Could you check a few things on this model? Use its own coordinates, in mm. Face numbers are marked on the shaded views. Round coordinates to 2 decimals unless told otherwise and drop trailing zeros. Write each loop counter-clockwise with the first axis right and the second up, starting at its lowest first coordinate (ties: lowest second). Pieces come first, ordered by that corner, then holes. Notation, with made-up numbers: (19.5, 44) - (44.5, 44) arc R23 ccw to (44.5, 75) - close; hole circle Ø4 at (2, -33.75). An arc over 180 degrees is marked (long way). Put each result on its own line as item: value.
from build123d import *

# Parameters (mm, degrees)
SKETCH1_W           = 101.6
SKETCH1_H           = 381
BOSS_EXTRUDE1_DEPTH = 3.175
CHAMFER1_SIZE       = 3.175
CUT_EXTRUDE1_REACH  = 199.183
SKETCH2_R           = 23.981466634
SKETCH2_R_2         = 10.952088468
SKETCH2_R_3         = 9.996566117
SKETCH2_W           = 34.925
SKETCH2_H           = 132.842153018
CHAMFER2_SIZE       = 3.175
FILLET1_R           = 5
FILLET2_R           = 5


with BuildPart() as part:
    # Sketch1 → Boss-Extrude1 (new body)
    with BuildSketch(Plane(origin=(0, 0, 0), x_dir=(1, 0, 0), z_dir=(0, 1, 0))):
        Rectangle(SKETCH1_W, SKETCH1_H)
    extrude(amount=BOSS_EXTRUDE1_DEPTH)

    # Chamfer1
    chamfer1_edges = [part.edges().sort_by_distance(p)[0] for p in [
        (50.8, 1.5875, 190.5),
        (-50.8, 1.5875, 190.5),
        (-50.8, 1.5875, -190.5),
        (50.8, 1.5875, -190.5),
    ]]
    chamfer(chamfer1_edges, length=CHAMFER1_SIZE)

    # Sketch2 → Cut-Extrude1 (cut, up to next)
    with BuildSketch(Plane(origin=(0, 3.175, 0), x_dir=(1, 0, 0), z_dir=(0, 1, 0)), mode=Mode.PRIVATE) as cut_extrude1_sk1:
        with Locations((41.515832085, -168.095479014)):
            Circle(SKETCH2_R)
    cut_extrude1_tool1 = extrude(cut_extrude1_sk1.sketch, amount=-CUT_EXTRUDE1_REACH, mode=Mode.PRIVATE) & part.part
    # Sketch2 → Cut-Extrude1 (cut, up to next)
    with BuildSketch(Plane(origin=(0, 3.175, 0), x_dir=(1, 0, 0), z_dir=(0, 1, 0)), mode=Mode.PRIVATE) as cut_extrude1_sk2:
        with Locations(Location((1.89865, 162.0774, 0), (0, 0, 270))):
            Circle(SKETCH2_R_2)
    cut_extrude1_tool2 = extrude(cut_extrude1_sk2.sketch, amount=-CUT_EXTRUDE1_REACH, mode=Mode.PRIVATE) & part.part
    # Sketch2 → Cut-Extrude1 (cut, up to next)
    with BuildSketch(Plane(origin=(0, 3.175, 0), x_dir=(1, 0, 0), z_dir=(0, 1, 0)), mode=Mode.PRIVATE) as cut_extrude1_sk3:
        with Locations(Location((1.89865, 88.265, 0), (0, 0, 270))):
            Circle(SKETCH2_R_3)
    cut_extrude1_tool3 = extrude(cut_extrude1_sk3.sketch, amount=-CUT_EXTRUDE1_REACH, mode=Mode.PRIVATE) & part.part
    # Sketch2 → Cut-Extrude1 (cut, up to next)
    with BuildSketch(Plane(origin=(0, 3.175, 0), x_dir=(1, 0, 0), z_dir=(0, 1, 0)), mode=Mode.PRIVATE) as cut_extrude1_sk4:
        with Locations((33.3375, 124.078923491)):
            Rectangle(SKETCH2_W, SKETCH2_H)
    cut_extrude1_tool4 = extrude(cut_extrude1_sk4.sketch, amount=-CUT_EXTRUDE1_REACH, mode=Mode.PRIVATE) & part.part
    add(cut_extrude1_tool1.solids().sort_by_distance((41.515832, 3.175, 168.095479))[0], mode=Mode.SUBTRACT)
    add(cut_extrude1_tool2.solids().sort_by_distance((1.89865, 3.175, -162.0774))[0], mode=Mode.SUBTRACT)
    add(cut_extrude1_tool3.solids().sort_by_distance((1.89865, 3.175, -88.265))[0], mode=Mode.SUBTRACT)
    add(cut_extrude1_tool4.solids().sort_by_distance((33.3375, 3.175, -124.078923))[0], mode=Mode.SUBTRACT)

    # Chamfer2
    chamfer2_edges = [part.edges().sort_by_distance(p)[0] for p in [
        (15.875, 1.5875, -190.5),
        (50.8, 1.5875, -57.657846982),
    ]]
    chamfer(chamfer2_edges, length=CHAMFER2_SIZE)

    # Fillet1
    fillet1_edges = [part.edges().sort_by_distance(p)[0] for p in [
        (15.875, 1.5875, -57.657846982),
    ]]
    fillet(fillet1_edges, radius=FILLET1_R)

    # Fillet2
    fillet2_edges = [part.edges().sort_by_distance(p)[0] for p in [
        (32.963161081, 1.5875, 190.5),
    ]]
    fillet(fillet2_edges, radius=FILLET2_R)


solid = part.part
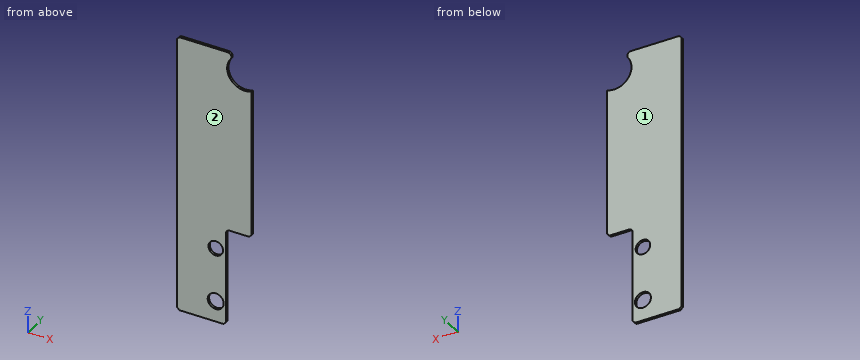
(1) If we mould it in two halves opening along Y, with no side actions, what happens to the marked faces 1 and 2? For each: pulls with the +Y half, pulls with the -Y half, needs draft (parallel to the pull), parting line crosses it, or undercut.
Values found:
face 1: pulls with the +Y half
face 2: pulls with the -Y half
(2) Imagine slicing it at B-B, the plane z = -133.5. List the corners of the cut face in (x, y) for me (3 decimals).
Values found:
outline: (-50.8, 0) - (15.875, 0) - (15.875, 3.175) - (-50.8, 3.175) - close
(3) Imagine slicing it at A-A, the plane y = 2.3. List the corners of the cut face in (x, z) for me (3 decimals), then the cut area to 3 significant figures.
Values found:
outline: (-50.8, -187.325) - (-47.625, -190.5) - (12.7, -190.5) - (15.875, -187.325) - (15.875, -62.658) arc R5 cw to (20.875, -57.658) - (47.625, -57.658) - (50.8, -54.483) - (50.8, 145.984) arc R23.981 cw to (22.34, 182.497) arc R5 ccw to (18.342, 190.5) - (-47.625, 190.5) - (-50.8, 187.325) - close; hole circle Ø21.904 at (1.899, -162.077); hole circle Ø19.993 at (1.899, -88.265)
area: 32,000 mm^2
(4) Please list where these lines run through material, in increasing order: probe 1 along Z at (x, y) = (1, 2.8); probe 2 along Z at (x, y) = (0, 2.95); probe 3 along X at (y, z) = (0.45, -162.5) (3 decimals). Write a range as from..to.
Values found:
probe 1: z = -190.5..-172.99, -151.16..-98.22, -78.31..190.5
probe 2: z = -190.5..-172.86, -151.29..-98.08, -78.45..190.5
probe 3: x = -50.8..-9.045, 12.843..15.875
(5) Imagine slicing it at C-C, the plane x = 30. List the corners of the cut face in (y, z) for me (3 decimals).
Values found:
outline: (0, -57.658) - (3.175, -57.658) - (3.175, 147.06) - (0, 147.06) - close
(6) I'm going to push flat-ended pins straight in: pin 1 (13 mm diameter, centred on x = 1.9, z = -162.08, fed in from +Y); pin 2 (1 mm diameter, centred on x = 22, y = 0.5, fed in from +Z). Where does each tip first touch, or does it pass through?
Values found:
pin 1: passes through
pin 2: stops at z = 189.38
